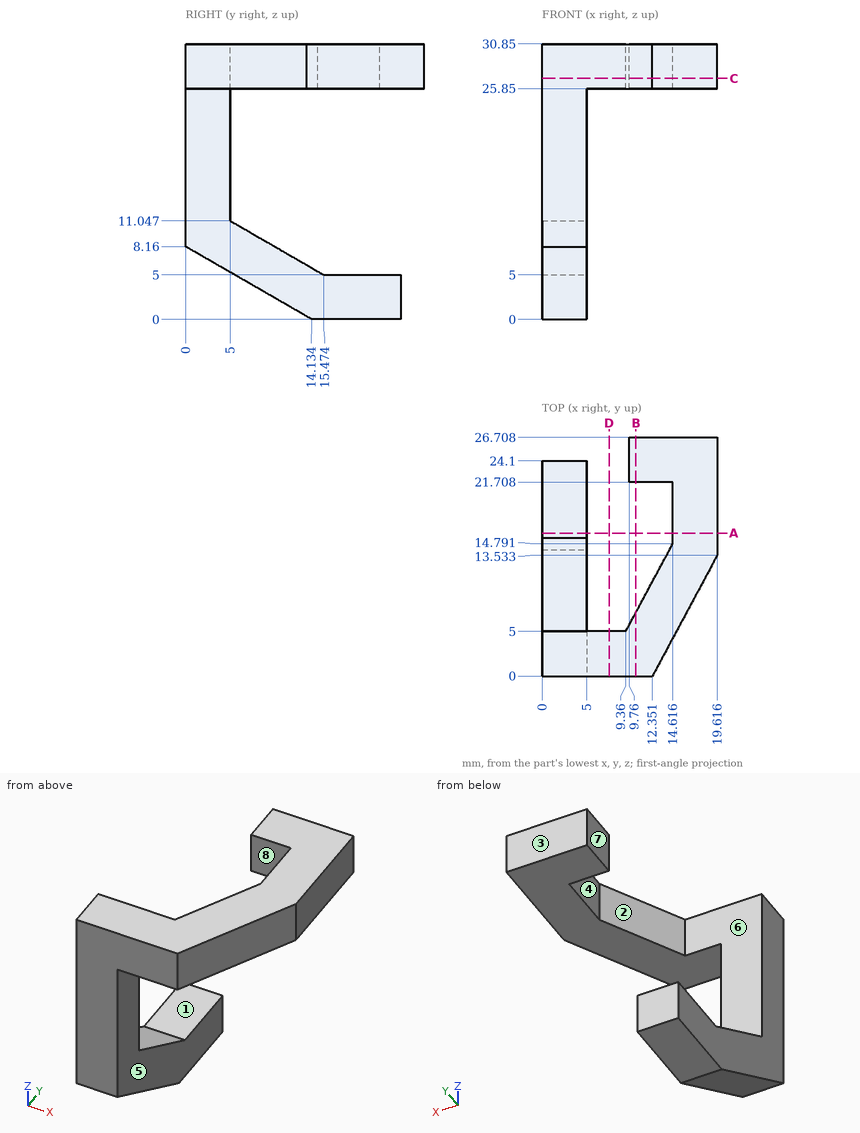
Answer from the drawing. Dimensions are ordinates in mm from the lowest x, y and z of the part. A direction names the side the tool comes from. Round coordinates to 2 decimals unless told otherwise and drop trailing zeros. Write each loop counter-clockwise with the first axis right and the second up, starting at its lowest first coordinate (ties: lowest second). Pieces come first, ordered by that corner, then holes. Notation, with made-up numbers: (-38.75, -18) -> (17.25, -18) arc R22 ccw to (17.25, 4) -> close; hole circle Ø3 at (-25, -23). An arc over 180 degrees is marked (long way). Answer in a Markdown table with one row per item. Add a question column.
1) Find section B-B, the plane x = 10.5. Determine the outline of the cut face in (y, z).
2) Find section C-C, the plane z = 27. Determine the outline of the cut face in (x, y).
3) Determine the mould class of the marked faces 1, 2, 3 and 4 for opening direction Y: pulls with the +Y half, pulls with the -Y half, needs draft (parallel to the pull), parting line crosses it, or undercut.
4) Find section D-D, the plane x = 7.5. Determine the outline of the cut face in (y, z), and give its area (3 significant figures).
5) Find section A-A, the plane y = 16. Determine the outline of the cut face in (x, z).
6) Consider line 1 (X direction, y = 4.5, z = 6); line 2 (Z direction, x = 5.5, y = 2). Determine where each line is inside the solid, lowest interval first.
7) Given P1, Ø1.5, axis at x = 17, y = 22, coming from the -Z side; P2, Ø1.5, axis at x = 12.5, z = 29.5, coming from the -Y side; P3, Ø1.5, axis at y = 19, z = 27.5, coming from the -X side; P4, Ø10, axis at x = 7, z = 6, coming from the +Y side, each flat-ended and moving along its own axis, determine where each tip first touches the part or whether it passes through.
8) Which of the six approach directions +Z, -Z, +X, -X, +Y, -Y give full straight-line access (tool end or side, diameter ignored) to the marked faces 5, 6, 7 and 8?
Findings below:
| question | item | result |
|---|---|---|
| 1 | outline | (0, 25.85) -> (7.12, 25.85) -> (7.12, 30.85) -> (0, 30.85) -> close; (21.71, 25.85) -> (26.71, 25.85) -> (26.71, 30.85) -> (21.71, 30.85) -> close |
| 2 | outline | (0, 0) -> (12.35, 0) -> (19.62, 13.53) -> (19.62, 26.71) -> (9.76, 26.71) -> (9.76, 21.71) -> (14.62, 21.71) -> (14.62, 14.79) -> (9.36, 5) -> (0, 5) -> close |
| 3 | face 1 | needs draft |
| 3 | face 2 | undercut |
| 3 | face 3 | pulls with the +Y half |
| 3 | face 4 | undercut |
| 4 | outline | (0, 25.85) -> (5, 25.85) -> (5, 30.85) -> (0, 30.85) -> close |
| 4 | area | 25.0 mm² |
| 5 | outline | (0, 0) -> (5, 0) -> (5, 5) -> (0, 5) -> close; (14.62, 25.85) -> (19.62, 25.85) -> (19.62, 30.85) -> (14.62, 30.85) -> close |
| 6 | line 1 | 0 to 5 |
| 6 | line 2 | 25.85 to 30.85 |
| 7 | P1 | z = 25.85 |
| 7 | P2 | y = 0 |
| 7 | P3 | x = 14.62 |
| 7 | P4 | y = 24.1 |
| 8 | face 5 | -Z, +X, +Y, -Y |
| 8 | face 6 | +Z, -X, +Y |
| 8 | face 7 | +Z, -Z, -X, +Y |
| 8 | face 8 | +Z, -Z, -X |
